Job drawing, mm, ordinate dimensions from the low corner. One solid piece. A direction names the side the tool comes from. Give positions to 0.01 mm unless a question says otherwise; leave off trailing zeros. Order: outer loops, then holes, each group sorted by start corner. A loop starts at its lowest first (then second) coordinate and runs counter-clockwise, first axis right, second up. Notation, with made-up numbers: M 83.25,2.25 L 101.25,2.25 A19 cw 101.25,6.25 Z; hole C 31.5,-6 d9. An arc over 180 degrees is marked long. One line per question, with ' | ' between items.
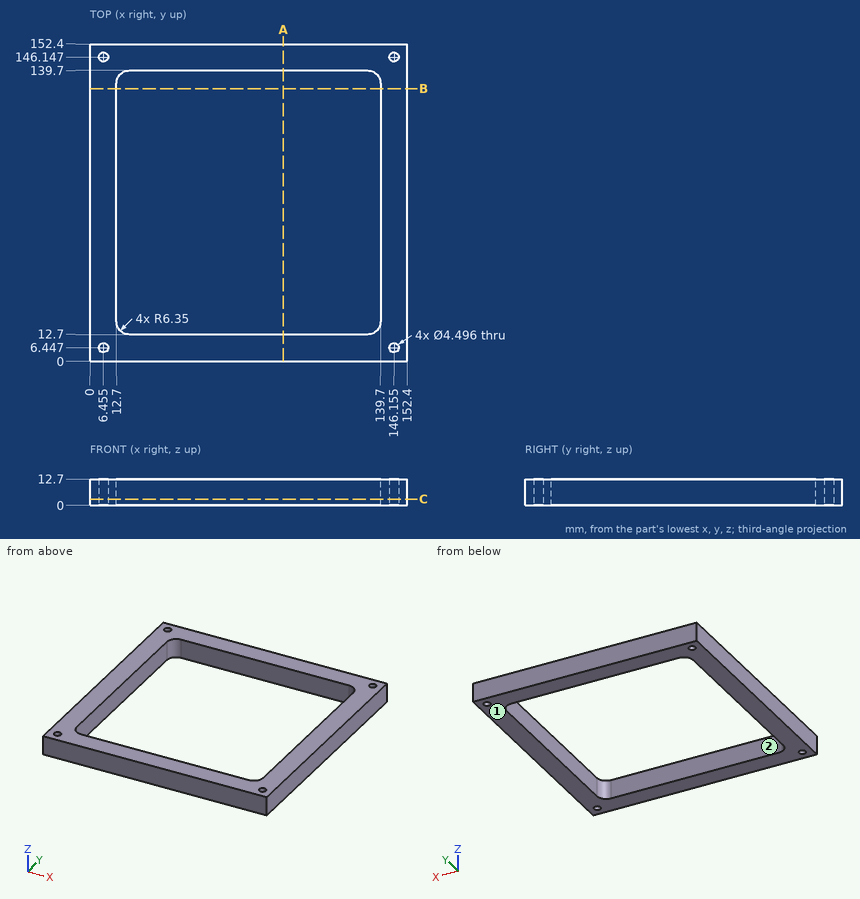
1. Slice it at A-A on x = 93. Give the cut face in (y, z).
Worked out:
outline: M 0,0 L 12.7,0 L 12.7,12.7 L 0,12.7 Z; M 139.7,0 L 152.4,0 L 152.4,12.7 L 139.7,12.7 Z
2. Tool access for the marked faces 1 and 2: list every direction of +Z, -Z, +X, -X, +Y, -Y with a clear straight run to the whole face (end or side of a thin tool).
Worked out:
face 1: -Z, +X, -X, +Y, -Y | face 2: +Z, -Z
3. Probe L1, parallel to Y at x = 146, z = 9.25 (1 decimal); L2, parallel to Y at x = 118, z = 2. List the from-to ranges inside material, lowest first. Write a range as from..to.
Worked out:
L1: y = 0..4.2, 8.7..143.9, 148.4..152.4 | L2: y = 0..12.7, 139.7..152.4
4. Slice it at C-C on z = 3. Give the number of separate pieces and of enclosed holes in the cut face, then the cut area to 3 significant figures.
Worked out:
separate pieces: 1 | enclosed holes: 5 | area: 7,070 mm2
5. Drop a flat-ended pin along its axis: pin 1 (2.5 mm diameter, centred on x = 6.45, y = 146.15, fed in from +Z). Give the stop position or say it passes through.
Worked out:
pin 1: passes through
